Drawing for the job (mm, zero at the part's lowest x, y, z). A direction names the side the tool comes from. Give positions to 0.01 mm unless a question says otherwise; leave off trailing zeros. Order: outer loops, then holes, each group sorted by start corner. A loop starts at its lowest first (then second) coordinate and runs counter-clockwise, first axis right, second up. Notation, with made-up numbers: (-25, -3.75) - (16, -3.75) arc R24 ccw to (16, 23.25) - close; hole circle Ø3 at (-4, -16). An arc over 180 degrees is marked (long way). Use CSV: the item, a comma, the result in double quotes. Start each with the question number.
(1) Drop flat-ended pins along their axis: pin 1 Ø6 at (x, y) = (98.5, 130) entering from +Z; pin 2 Ø2.5 at (x, z) = (10, 4.5) entering from -Y; pin 3 Ø1.5 at (y, z) = (26, 5) entering from -X; pin 4 Ø4 at (x, y) = (125, 10) entering from -Z. Give the stop position or say it passes through.
(2) Probe L1, parallel to Y at x = 40, z = 1.8; L2, parallel to Y at x = 125, z = 4.5; L3, parallel to Y at x = 78.5, z = 3.4. List the from-to ranges inside material, lowest first.
(3) Band-saw the part on B-B, the plane y = 10. Give the cut face in (x, z).
(4) Band-saw the part on D-D, the plane x = 66.5. Give the cut face in (y, z).
(5) Band-saw the part on C-C, the plane z = 3.9. Give the cut face in (x, y), then the cut area to 3 significant figures.
(6) Tool access for the marked faces 1, 2 and 3: list every direction of +Z, -Z, +X, -X, +Y, -Y with a clear straight run to the whole face (end or side of a thin tool).
(7) Band-saw the part on A-A, the plane x = 40. Give the cut face in (y, z).
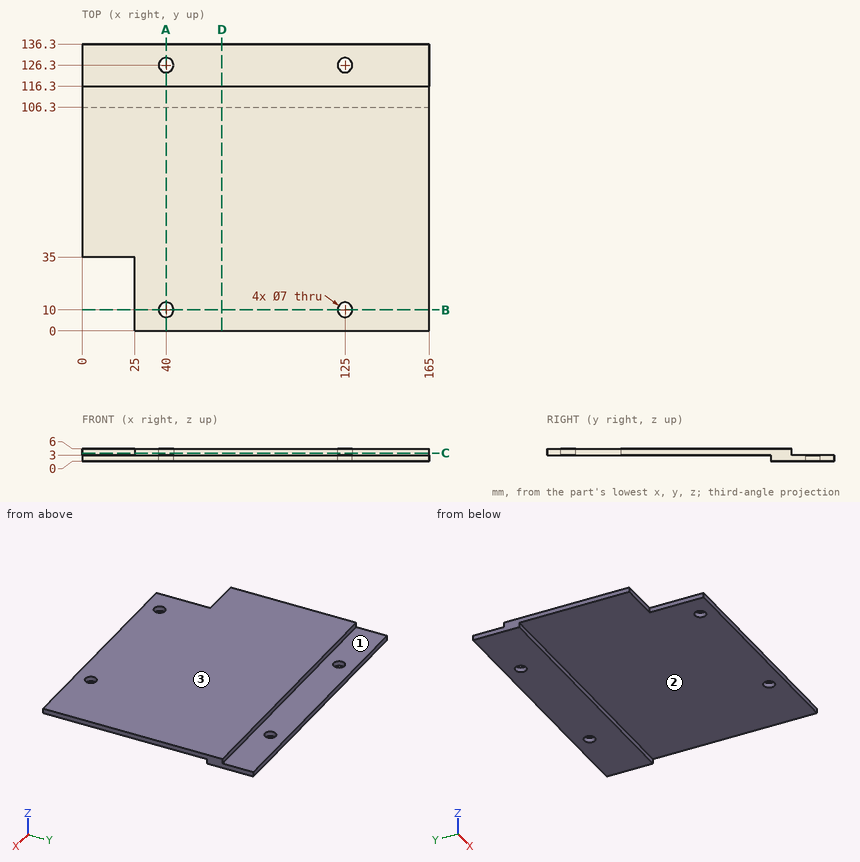
Answer block:
1,pin 1,"stops at z = 3"
1,pin 2,"stops at y = 35"
1,pin 3,"stops at x = 25"
1,pin 4,"passes through"
2,L1,"y = 106.3 to 122.8, 129.8 to 136.3"
2,L2,"y = 0 to 6.5, 13.5 to 116.3"
2,L3,"y = 0 to 116.3"
3,outline,"(25, 3) - (36.5, 3) - (36.5, 6) - (25, 6) - close; (43.5, 3) - (121.5, 3) - (121.5, 6) - (43.5, 6) - close; (128.5, 3) - (165, 3) - (165, 6) - (128.5, 6) - close"
4,outline,"(0, 3) - (106.3, 3) - (106.3, 0) - (136.3, 0) - (136.3, 3) - (116.3, 3) - (116.3, 6) - (0, 6) - close"
5,outline,"(0, 35) - (25, 35) - (25, 0) - (165, 0) - (165, 116.3) - (0, 116.3) - close; hole circle Ø7 at (40, 10); hole circle Ø7 at (125, 10)"
5,area,"18,200 mm2"
6,face 1,"+Z, +X, -X, +Y"
6,face 2,"-Z, +X, -X, -Y"
6,face 3,"+Z, +X, -X, +Y, -Y"
7,outline,"(0, 3) - (6.5, 3) - (6.5, 6) - (0, 6) - close; (13.5, 3) - (106.3, 3) - (106.3, 0) - (122.8, 0) - (122.8, 3) - (116.3, 3) - (116.3, 6) - (13.5, 6) - close; (129.8, 0) - (136.3, 0) - (136.3, 3) - (129.8, 3) - close"
